from build123d import *

# Parameters (mm, degrees)
F2_R      = 0.508
F4_DEPTH  = 25.401
F5_R      = 0.635
F6_DEPTH  = 13.330517
F7_R      = 0.635
F8_DEPTH  = 3.81
F10_DEPTH = 25.401


with BuildPart() as f1:
    # F0 (on Right) → F1 (revolve)
    with BuildSketch(Plane.YZ):
        with BuildLine():
            Line((-25.4, 1), (0, 1))
            Line((0, 1), (0, 12.7))
            ThreePointArc((0, 12.7), (-1.27, 13.329516), (-2.54, 12.7))
            Line((-2.54, 12.7), (-3.699565, 11.176))
            Line((-3.699565, 11.176), (-4.969565, 11.176))
            Line((-4.969565, 11.176), (-4.969565, 12.7))
            Line((-4.969565, 12.7), (-12.7, 2.54))
            Line((-12.7, 2.54), (-25.4, 2.54))
            Line((-25.4, 2.54), (-25.4, 1))
        make_face()
    revolve(axis=Axis((0, -12.7, 0), (0, -1, 0)))

    # F2
    f2_edges = [f1.edges().sort_by_distance(p)[0] for p in [
        (0, -4.969565, -12.7),
    ]]
    fillet(f2_edges, radius=F2_R)

    # F3 (on face) → F4 (cut, through all)
    with BuildSketch(Plane(origin=(0, 0, 0), x_dir=(-1, 0, 0), z_dir=(0, 1, 0))):
        with BuildLine():
            ThreePointArc((-1.143, 0.127), (-1.27, 0), (-1.143, -0.127))
            Line((-1.143, -0.127), (1.143, -0.127))
            ThreePointArc((1.143, -0.127), (1.27, 0), (1.143, 0.127))
            Line((1.143, 0.127), (-1.143, 0.127))
        make_face()
    extrude(amount=-F4_DEPTH, mode=Mode.SUBTRACT)

    # F5 (on Right) → F6 (cut, through all)
    with BuildSketch(Plane.YZ):
        with Locations((-4.334565, 0)):
            Circle(F5_R)
    extrude(amount=-F6_DEPTH, mode=Mode.SUBTRACT)

    # F7 (on face) → F8 (cut)
    with BuildSketch(Plane(origin=(0, 0, 0), x_dir=(-1, 0, 0), z_dir=(0, 1, 0))):
        with Locations((11.43, -2.54)):
            Circle(F7_R)
    extrude(amount=-F8_DEPTH, mode=Mode.SUBTRACT)

    # F9 (on face) → F10 (cut, through all)
    with BuildSketch(Plane(origin=(0, 0, 0), x_dir=(-1, 0, 0), z_dir=(0, 1, 0))):
        with BuildLine():
            ThreePointArc((-1.19589, 0.377311), (-1.524, 0), (-1.19589, -0.377311))
            ThreePointArc((-1.19589, -0.377311), (0, -1.254), (1.19589, -0.377311))
            ThreePointArc((1.19589, -0.377311), (1.524, 0), (1.19589, 0.377311))
            ThreePointArc((1.19589, 0.377311), (0, 1.254), (-1.19589, 0.377311))
        make_face()
        with BuildLine():
            Line((-1.143, 0.127), (-0.991903, 0.127))
            ThreePointArc((-0.991903, 0.127), (0, 1), (0.991903, 0.127))
            Line((0.991903, 0.127), (1.143, 0.127))
            ThreePointArc((1.143, 0.127), (1.27, 0), (1.143, -0.127))
            Line((1.143, -0.127), (0.991903, -0.127))
            ThreePointArc((0.991903, -0.127), (0, -1), (-0.991903, -0.127))
            Line((-0.991903, -0.127), (-1.143, -0.127))
            ThreePointArc((-1.143, -0.127), (-1.27, 0), (-1.143, 0.127))
        make_face(mode=Mode.SUBTRACT)
    extrude(amount=-F10_DEPTH, mode=Mode.SUBTRACT)


solid = f1.part
The listing builds one solid part. Answer for the finished solid, in the listing's coordinates (mm). A direction names the side the tool comes from. Coordinates: 2 decimals unless noted, no trailing zeros. Order: outer loops, then holes, each group sorted by start corner. A loop starts at its lowest first (then second) coordinate and runs counter-clockwise, first axis right, second up.
Q1. Which of the six approach directions +Z, -Z, +X, -X, +Y, -Y give full straight-line access (tool end or side, diameter ignored) to faces 4 (the face through (-2.52, -19.14, -0.33)), 5 (the face through (6.8, -4.34, -8.87)), 6 (the face through (0.022, -12.522, -1.254)), 7 (the face through (3, 0, 0)), 8 (the face through (1, -25.4, -1))?
Q2. A cutting plane is placed at C-C, the plane y = -10.5. Write down the section's boundary in (x, z).
Q3. Consider line 1 (X direction, y = -2.3, z = -2.54) (3 decimals); line 2 (Y direction, x = -3.75, z = 0); line 3 (Z direction, x = -11.43, y = -1.25) (3 decimals). Determine where each line is inside the solid, lowest interval first.
Q4. A cutting plane is placed at B-B, the plane y = -20.5. Write down the section's boundary in (x, z), and give its area (3 significant figures).
Q5. Given P1, Ø3, axis at x = -3.5, y = -13, coming from the -Z side; P2, Ø12, axis at y = -15.5, z = -7.5, coming from the -X side; P3, Ø8, axis at y = -11.5, z = 2.5, coming from the -X side, each flat-ended and moving along its own axis, determine where each tip first touches the part or whether it passes through.
Q6. For a pull along Y with two mould halves and no side action, classify faces 1 (the face through (1.81, -12.37, -2.36)), 2 (the face through (-6.06, -3.73, 0.19)), 3 (the face through (-10.796, -1.455, -2.512)) as pulls with the +Y half, pulls with the -Y half, needs draft (parallel to the pull), parting line crosses it, or undercut.
Answers follow:
1. face 4: -Y
1. face 5: none
1. face 6: +Y, -Y
1. face 7: +Z, -Z, +X, -X, +Y
1. face 8: +Z, -Z, +X, -X, -Y
2. outline: circle Ø10.86 at (0, 0); hole (-1.2, -0.38) arc R1.25 ccw to (1.2, -0.38) arc R0.38 ccw to (1.2, 0.38) arc R1.25 ccw to (-1.2, 0.38) arc R0.38 ccw to start
3. line 1: x = -12.701 to -12.065, -10.795 to 12.701
3. line 2: y = -11.78 to -4.97, -3.7 to 0
3. line 3: z = -6.858 to -3.175, -1.905 to 6.858
4. outline: circle Ø5.08 at (0, 0); hole (-1.2, -0.38) arc R1.25 ccw to (1.2, -0.38) arc R0.38 ccw to (1.2, 0.38) arc R1.25 ccw to (-1.2, 0.38) arc R0.38 ccw to start
4. area: 15.0 mm2
5. P1: stops at z = -2.7
5. P2: stops at x = -3.48
5. P3: stops at x = -9.12
6. face 1: pulls with the -Y half
6. face 2: undercut
6. face 3: needs draft
